Autodesk Inventor part; units mm, degrees
ref_plane "YZ Plane" through (0, 0, 0) normal (1, 0, 0) x (0, 1, 0)
ref_plane "XZ Plane" through (0, 0, 0) normal (0, 1, 0) x (-1, 0, 0)
ref_plane "XY Plane" through (0, 0, 0) normal (0, 0, 1) x (1, 0, 0)
sketch "Sketch1" plane through (0, 0, 0) normal (0, 0, 1) x (1, 0, 0)
  circle A0 centre (0, 0) radius 10.16
  arc A1 (-0.762, 3.0822) -> (0.762, 3.0822) centre (0, 0) ccw
  line L0 (0.762, 3.0822) -> (0.762, 3.8442)
  line L1 (0.762, 3.8442) -> (-0.762, 3.8442)
  line L2 (-0.762, 3.8442) -> (-0.762, 3.0822)
  point P0 (0, 3.0822)
extrude "Extrusion1" add sketch "Sketch1" along normal blind 12.7
sketch "Sketch2" plane through (0, 0, 12.7) normal (0, 0, 1) x (1, 0, 0)
  arc A0 (0.8854, 14.7054) -> (-0.8926, 14.7049) centre (0, 0) ccw
  arc A1 (-0.762, 3.0822) -> (0.762, 3.0822) centre (0, 0) ccw
  circle A2 centre (0, 0) radius 10.16
  arc A3 (1.5168, 10.0461) -> (0.8854, 14.7054) centre (-8.8522, 11.0133) ccw
  arc A4 (-0.8926, 14.7049) -> (-1.524, 10.045) centre (8.8449, 11.0129) ccw
  dimension "d6" = 29.464
  dimension "d8" = 10.414
  dimension "d9" = 10.414
  dimension "d12" = 1.778
extrude "Extrusion2" add sketch "Sketch2" against normal blind 12.7 contours A3 A2 A4 A0
pattern_circular "Circular Pattern1" count 12 over 360 about axis through (0, 0, 0) along (0, 0, 1) of "Extrusion2"
properties part number "Gear" material "Stainless Steel"
Can you work these out from the model? Positions are in its coordinate system, mm. A direction names the side the tool comes from. Give positions to 0.01 mm unless a question says otherwise; leave off trailing zeros. Loops run counter-clockwise (first coordinate to the right, second up) from the corner with the lowest first, then second, coordinate; pieces in that order, holes last. Notation, with made-up numbers: (51.25, 86) - (66.25, 86) arc R12 ccw to (66.25, 91) - close; hole circle Ø11 at (13, -37). An arc over 180 degrees is marked (long way). Answer as a JSON object with one key per item and string values.
Q1. Which directions (+Z, -Z, +X, -X, +Y, -Y) give clear straight access to the entire face, cutting with the end or side of a thin tool? Please do faces 1 (the cylindrical face through (11.456, 4.915, 6.439)), 2 (the cylindrical face through (7.374, 12.754, 6.439)), 3 (the cylindrical face through (-4.915, 11.456, 6.439)), 4 (the cylindrical face through (-12.38, 1.47, 6.44)).
Geometry says:
{"face 1": "+Z, -Z, +X", "face 2": "+Z, -Z, +X, +Y", "face 3": "+Z, -Z, +Y", "face 4": "+Z, -Z"}
Q2. Imagine slicing it at A-A on y = 0. Write out the boundary of the cut face in (x, z) (3 decimals).
Geometry says:
{"outline": "(-14.732, 0) - (-3.175, 0) - (-3.175, 12.7) - (-14.732, 12.7) - close; (3.175, 0) - (14.732, 0) - (14.732, 12.7) - (3.175, 12.7) - close"}
Q3. Imagine slicing it at B-B on x = 0. Write out the boundary of the cut face in (y, z) (3 decimals), plus the area to 3 significant figures.
Geometry says:
{"outline": "(-14.732, 0) - (-3.175, 0) - (-3.175, 12.7) - (-14.732, 12.7) - close; (3.844, 0) - (14.732, 0) - (14.732, 12.7) - (3.844, 12.7) - close", "area": "285 mm²"}
Q4. If I drill on L1, parallel to X at y = 0, z = 7.75 (3 decimals); L2, parallel to X at y = -7.25, z = 3.25; L3, parallel to X at y = -12.75, z = 3, over which ranges is the centre line in solid material (lowest first)?
Geometry says:
{"L1": "-14.732 to -3.175, 3.175 to 14.732", "L2": "-12.82 to -9.48, -7.12 to 7.12, 9.5 to 12.82", "L3": "-7.38 to -6.08, -1.42 to 1.42, 6.09 to 7.38"}
Q5. If we mould it in two halves opening along Y, with no side actions, what happens to faces 5 (the cylindrical face through (7.2, -7.17, 6.26)), 6 (the cylindrical face through (-7.374, -12.754, 6.439)), 7 (the cylindrical face through (-7.36, 12.76, 6.44))? For each: pulls with the +Y half, pulls with the -Y half, needs draft (parallel to the pull), parting line crosses it, or undercut.
Geometry says:
{"face 5": "undercut", "face 6": "pulls with the -Y half", "face 7": "pulls with the +Y half"}
Q6. Imagine slicing it at D-D on y = -10.75. Write out the boundary of the cut face in (x, z).
Geometry says:
{"outline": "(-7.75, 0) - (-4.41, 0) - (-4.41, 12.7) - (-7.75, 12.7) - close; (-1.56, 0) - (1.57, 0) - (1.57, 12.7) - (-1.56, 12.7) - close; (4.42, 0) - (7.75, 0) - (7.75, 12.7) - (4.42, 12.7) - close"}
Q7. Will these pins go through, and if not, where does the flat tip stop? P1, Ø5, axis at x = 8.5, z = 8.5, coming from the +Y side; P2, Ø1, axis at y = -5.5, z = 7.5, coming from the -X side; P3, Ø1.5, axis at y = -3, z = 10, coming from the -X side; P4, Ø4, axis at x = 0, y = 0, coming from the +Z side.
Geometry says:
{"P1": "y = 13.18", "P2": "x = -12.66", "P3": "x = -9.91", "P4": "through"}
Q8. Imagine slicing it at C-C on x = -10.5. Write out the boundary of the cut face in (y, z), plus the area to 3 significant figures.
Geometry says:
{"outline": "(-7.67, 0) - (-4.26, 0) - (-4.26, 12.7) - (-7.67, 12.7) - close; (-1.56, 0) - (1.55, 0) - (1.55, 12.7) - (-1.56, 12.7) - close; (4.25, 0) - (7.66, 0) - (7.66, 12.7) - (4.25, 12.7) - close", "area": "126 mm²"}
